Autodesk Inventor part; units mm, degrees
ref_plane "YZ Plane" through (0, 0, 0) normal (1, 0, 0) x (0, 1, 0)
ref_plane "XZ Plane" through (0, 0, 0) normal (0, 1, 0) x (-1, 0, 0)
ref_plane "XY Plane" through (0, 0, 0) normal (0, 0, 1) x (1, 0, 0)
sketch "Sketch1" plane through (0, 0, 0) normal (0, 0, 1) x (1, 0, 0)
  line L0 (0, 0) -> (0, 10)
  line L1 (0, 10) -> (188, 10)
  line L2 (188, 10) -> (188, 7.5)
  line L3 (188, 7.5) -> (195, 7.5)
  line L4 (195, 7.5) -> (195, 7.5)
  line L5 (195, 7.5) -> (217, 7.5)
  line L6 (265, 0) -> (0, 0)
  line L7 (217, 7.5) -> (217, 6)
  line L8 (217, 6) -> (265, 6)
  line L9 (265, 6) -> (265, 0)
  line L10 (0, 10) -> (-188, 10)
  line L11 (-188, 10) -> (-188, 7.5)
  line L12 (-188, 7.5) -> (-195, 7.5)
  line L13 (-195, 7.5) -> (-195, 7.5)
  line L14 (-195, 7.5) -> (-217, 7.5)
  line L15 (-265, 0) -> (0, 0)
  line L16 (-217, 7.5) -> (-217, 6)
  line L17 (-217, 6) -> (-265, 6)
  line L18 (-265, 6) -> (-265, 0)
  point P0 (188, 8.75)
  point P1 (217, 6.75)
  point P2 (-188, 8.75)
  point P3 (-217, 6.75)
  dimension "d0" = 10
  dimension "d1" = 188
  dimension "d2" = 7
  dimension "d4" = 265
  dimension "d5" = 6
  dimension "d6" = 7.5
  dimension "d7" = 7.5
  dimension "d12" = 217
revolve "Revolution1" add sketch "Sketch1" angle 360 about axis through (265, 0, 0) along (-1, 0, 0)
chamfer "Chamfer1" distance 1 angle 45 2 edges at (188, -10, 0) (-188, -10, 0)
thread "Thread1"
thread "Thread2"
sketch "Sketch3" plane through (-265, 0, 0) normal (-1, 0, 0) x (0, 0, 1)
  point P0 (0, 0)
  point P1 (0, 0)
hole "Hole1" at (-265, 0, 0) direction (1, 0, 0) diameter 4.917 depth 17.1 tip angle 118
sketch "Sketch4" plane through (265, 0, 0) normal (1, 0, 0) x (0, 0, -1)
  point P0 (0, 0)
  point P1 (0, 0)
hole "Hole2" at (265, 0, 0) direction (-1, 0, 0) diameter 4.917 depth 17.1 tip angle 118
properties part number "P301" material "Steel, Mild"
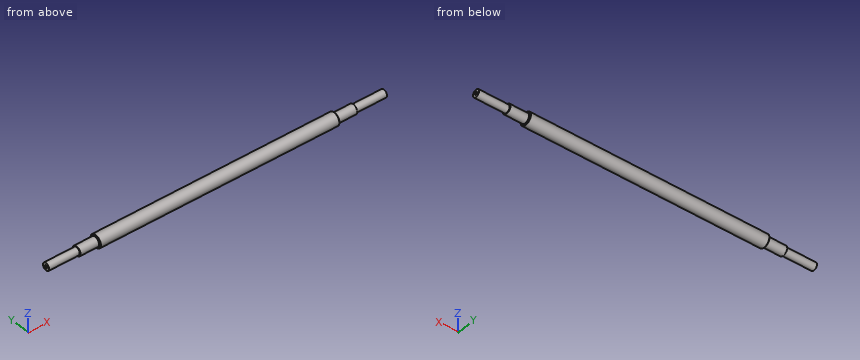
Input: part model. Units: mm. Frame: model coordinates. Coordinates: 2 decimals unless noted, no trailing zeros. Order: outer loops, then holes, each group sorted by start corner. A loop starts at its lowest first (then second) coordinate and runs counter-clockwise, first axis right, second up. Notation, with made-up numbers: (9, 75) - (27, 75) arc R23 ccw to (27, 87) - close; hole circle Ø1 at (41, -18). An arc over 180 degrees is marked (long way). Return JSON: item names as keys, results as strings.
Q1. First-contact query: pin 1 (10 mm diameter, centred on x = 65, y = -3.5, fed in from -Z); pin 2 (8 mm diameter, centred on x = 86, y = 8, fed in from +Z); pin 3 (3 mm diameter, centred on y = 0, z = 0, fed in from +X); pin 4 (6 mm diameter, centred on x = -65.5, z = -5.5, fed in from -Y). Flat tips, straight axial feed; report the tip coordinate or a pass-through.
The answers:
{"pin 1": "stops at z = -10", "pin 2": "stops at z = 9.17", "pin 3": "stops at x = 247.32", "pin 4": "stops at y = -9.68"}
Q2. Cut plane A-A (x = 29). Return loops of the section in (y, z), then the cut area to 3 significant figures.
The answers:
{"outline": "circle Ø20 at (0, 0)", "area": "314 mm2"}
Q3. Ray query, probe 1 along Y at (x, z) = (-257.5, 0); probe 2 along Z at (x, y) = (-25, -0.75). Return the intervals inside material, ascending.
The answers:
{"probe 1": "y = -6 to -2.46, 2.46 to 6", "probe 2": "z = -9.97 to 9.97"}
